```python
from build123d import *

# Parameters (mm, degrees)
ESQUISSE1_R             = 39
ESQUISSE1_R_2           = 16.175
BOSS_EXTRU_1_DEPTH      = 5
ESQUISSE2_R             = 49
BOSS_EXTRU_2_DEPTH      = 5
ESQUISSE3_R             = 16.175
ENL_V_MAT_EXTRU_1_DEPTH = 11
ESQUISSE4_R             = 1.5
ESQUISSE4_R_2           = 5
ENL_V_MAT_EXTRU_2_DEPTH = 11


with BuildPart() as part:
    # Esquisse1 → Boss.-Extru.1 (new body)
    with BuildSketch(Plane.XY):
        Circle(ESQUISSE1_R)
        Circle(ESQUISSE1_R_2, mode=Mode.SUBTRACT)
    extrude(amount=BOSS_EXTRU_1_DEPTH)

    # Esquisse2 → Boss.-Extru.2 (add)
    with BuildSketch(Plane(origin=(0, 0, 0), x_dir=(-1, 0, 0), z_dir=(0, 0, -1))):
        Circle(ESQUISSE2_R)
    extrude(amount=BOSS_EXTRU_2_DEPTH)

    # Esquisse3 → Enlèv. mat.-Extru.1 (cut, through all)
    with BuildSketch(Plane(origin=(0, 0, -5), x_dir=(-1, 0, 0), z_dir=(0, 0, -1))):
        Circle(ESQUISSE3_R)
    extrude(amount=-ENL_V_MAT_EXTRU_1_DEPTH, mode=Mode.SUBTRACT)

    # Esquisse4 → Enlèv. mat.-Extru.2 (cut, through all)
    with BuildSketch(Plane(origin=(0, 0, -5), x_dir=(-1, 0, 0), z_dir=(0, 0, -1))):
        with Locations((0, 44)):
            Circle(ESQUISSE4_R)
        with Locations((0, -44)):
            Circle(ESQUISSE4_R)
        with Locations((25, 0)):
            Circle(ESQUISSE4_R_2)
        with Locations((0, 25)):
            Circle(ESQUISSE4_R_2)
        with Locations((-25, 0)):
            Circle(ESQUISSE4_R_2)
        with Locations((0, -25)):
            Circle(ESQUISSE4_R_2)
        with Locations((-17.67766953, -17.67766953)):
            Circle(ESQUISSE4_R_2)
        with Locations((17.67766953, 17.67766953)):
            Circle(ESQUISSE4_R_2)
        with Locations((17.67766953, -17.67766953)):
            Circle(ESQUISSE4_R_2)
        with Locations((-17.67766953, 17.67766953)):
            Circle(ESQUISSE4_R_2)
    extrude(amount=-ENL_V_MAT_EXTRU_2_DEPTH, mode=Mode.SUBTRACT)


solid = part.part
```
Build history of the part. All positions in model axes, mm. A direction names the side the tool comes from. Give positions to 0.01 mm unless a question says otherwise; leave off trailing zeros. Order: outer loops, then holes, each group sorted by start corner. A loop starts at its lowest first (then second) coordinate and runs counter-clockwise, first axis right, second up. Notation, with made-up numbers: M 37.25,80.5 L 85.25,80.5 A19 cw 85.25,94.5 Z; hole C 87.5,17.25 d11. An arc over 180 degrees is marked long. Return JSON: item names as keys, results as strings.
Q1. Band-saw the part on D-D (x = -25). Give the cut face in (y, z).
Answer list:
{"outline": "M -42.14,-5 L -5,-5 L -5,5 L -29.93,5 L -29.93,0 L -42.14,0 Z; M 5,-5 L 42.14,-5 L 42.14,0 L 29.93,0 L 29.93,5 L 5,5 Z"}
Q2. 3-axis set-ups, long thin cutter, end or side, ignore diameter. For faces 1 (the face through (18.76, -22.56, -0.07)), 2 (the face through (15, 37, 0)): which of +Z, -Z, +X, -X, +Y, -Y reach the whole face in a straight line?
Answer list:
{"face 1": "+Z, -Z", "face 2": "+Z"}
Q3. Two-plate mould, pull along Y, no slides. Class faces 3 (the face through (-5.077, 38.668, 2.465)), 4 (the face through (0.325, -45.464, -2.535)), 5 (the face through (12, 12, -5)): pulls with the +Y half, pulls with the -Y half, needs draft (parallel to the pull), parting line crosses it, or undercut.
Answer list:
{"face 3": "parting line crosses it", "face 4": "undercut", "face 5": "needs draft"}
Q4. Wall check: probe 1 along Y at (x, z) = (0, 2.75) (3 decimals); probe 2 along X at (y, z) = (3.5, 3.25); probe 3 along Y at (x, z) = (-1.5, 3.5). Give the ranges that are in metal, low to high. Write a range as from..to.
Answer list:
{"probe 1": "y = -39..-30, -20..-16.175, 16.175..20, 30..39", "probe 2": "x = -38.84..-28.57, -21.43..-15.79, 15.79..21.43, 28.57..38.84", "probe 3": "y = -38.97..-29.77, -20.23..-16.11, 16.11..20.23, 29.77..38.97"}
Q5. Band-saw the part on C-C (z = -3.5). Count the separate pieces of the cut face and the enclosed holes in it, then the cut area to 3 significant figures.
Answer list:
{"separate pieces": "1", "enclosed holes": "11", "area": "6,080 mm^2"}
Q6. Flat gauge pins, fed straight in: pin 1 (2 mm diameter, centred on y = -35, z = 0.5, fed in from -X); pin 2 (1.5 mm diameter, centred on y = -29.5, z = -1.5, fed in from +X); pin 3 (5 mm diameter, centred on x = 0, y = -44, fed in from +Z). Where does each tip first touch, or does it go through?
Answer list:
{"pin 1": "stops at x = -35.15", "pin 2": "stops at x = 39.68", "pin 3": "stops at z = 0"}
Q7. Band-saw the part on B-B (y = 0). Give the cut face in (x, z) (3 decimals), then the cut area to 4 significant figures.
Answer list:
{"outline": "M -49,-5 L -30,-5 L -30,5 L -39,5 L -39,0 L -49,0 Z; M -20,-5 L -16.175,-5 L -16.175,5 L -20,5 Z; M 16.175,-5 L 20,-5 L 20,5 L 16.175,5 Z; M 30,-5 L 49,-5 L 49,0 L 39,0 L 39,5 L 30,5 Z", "area": "356.5 mm^2"}
Q8. Band-saw the part on A-A (x = 0). Give the cut face in (y, z) (3 decimals).
Answer list:
{"outline": "M -49,-5 L -45.5,-5 L -45.5,0 L -49,0 Z; M -42.5,-5 L -30,-5 L -30,5 L -39,5 L -39,0 L -42.5,0 Z; M -20,-5 L -16.175,-5 L -16.175,5 L -20,5 Z; M 16.175,-5 L 20,-5 L 20,5 L 16.175,5 Z; M 30,-5 L 42.5,-5 L 42.5,0 L 39,0 L 39,5 L 30,5 Z; M 45.5,-5 L 49,-5 L 49,0 L 45.5,0 Z"}
